from build123d import *

# Parameters (mm, degrees)
F0_W     = 25.4
F0_H     = 25.4
F1_DEPTH = 35.814
F1_TAPER = 19.471
F2_W     = 25.4
F2_H     = 25.4
F3_DEPTH = 35.814
F3_TAPER = 19.471


with BuildPart() as f1:
    # F0 (on Top) → F1 (new body)
    with BuildSketch(Plane.XY):
        Rectangle(F0_W, F0_H)
    extrude(amount=F1_DEPTH, taper=F1_TAPER)

    # F2 (on Top) → F3 (join)
    with BuildSketch(Plane.XY):
        Rectangle(F2_W, F2_H)
    extrude(amount=-F3_DEPTH, taper=F3_TAPER)


solid = f1.part
Could you check a few things on this model? Use its own coordinates, in mm. Round coordinates to 2 decimals unless told otherwise and drop trailing zeros. Write each loop counter-clockwise with the first axis right and the second up, starting at its lowest first coordinate (ties: lowest second). Pieces come first, ordered by that corner, then holes. Notation, with made-up numbers: (23, 66.5) - (42, 66.5) arc R22 cw to (42, 76.5) - close; hole circle Ø6 at (-7, 10.25). An arc over 180 degrees is marked (long way). Put each result on its own line as item: value. Start each with the question number.
(1) I need wall thicknesses on probe 1 along X at (y, z) = (4, -16.5); probe 2 along Y at (x, z) = (-6.5, -0.5). Which ranges of each line are inside material? Lowest first, please.
(2) Will these pins go through, and if not, where does the flat tip stop? pin 1 (5 mm diameter, centred on x = 1, z = 10.5, fed in from +Y); pin 2 (8 mm diameter, centred on x = 0.5, z = 11, fed in from +Y); pin 3 (1 mm diameter, centred on x = -5.5, z = -6, fed in from +Y).
(3) Thinking about a two-plate mould opening in X: for faces 1 (the flat face through (7.865, 0.178, 13.677)), 2 (the flat face through (-7.865, -0.178, 13.677)), 3 (the flat face through (-0.178, 7.865, 13.677)), which applies, released by +X, released by -X, zero draft, split by the parting line, or undercut?
(4) I want a section at A-A, the plane z = 1. Please give me the cut outline in (x, y), plus the area to 3 significant figures.
Here are the results:
1. probe 1: x = -6.87 to 6.87
1. probe 2: y = -12.52 to 12.52
2. pin 1: stops at y = 9.87
2. pin 2: stops at y = 10.23
2. pin 3: stops at y = 10.76
3. face 1: released by +X
3. face 2: released by -X
3. face 3: zero draft
4. outline: (-12.35, -12.35) - (12.35, -12.35) - (12.35, 12.35) - (-12.35, 12.35) - close
4. area: 610 mm^2
